Could you check a few things on this model? Use its own coordinates, in mm. A direction names the side the tool comes from. Coordinates: 2 decimals unless noted, no trailing zeros. Write each loop counter-clockwise with the first axis right and the second up, starting at its lowest first coordinate (ties: lowest second). Pieces come first, ordered by that corner, then holes. Notation, with made-up numbers: (-9.75, -6) - (44.25, -6) arc R28 ccw to (44.25, 12) - close; hole circle Ø2 at (2, 24.5). An arc over 180 degrees is marked (long way). Write item = value, one per line. Start each with the question number.
```python
from build123d import *

# Parameters (mm, degrees)
SKETCH1_W           = 57.5
SKETCH1_H           = 78
BOSS_EXTRUDE1_DEPTH = 30
SKETCH2_W           = 48.5
SKETCH2_H           = 26
CUT_EXTRUDE1_DEPTH  = 76
SKETCH3_R           = 2
SKETCH3_R_2         = 1
CUT_EXTRUDE2_DEPTH  = 60.424849114


with BuildPart() as part:
    # Sketch1 → Boss-Extrude1 (new body)
    with BuildSketch(Plane(origin=(0, 0, 0), x_dir=(1, 0, 0), z_dir=(0, 1, 0))):
        with Locations((-4.848039216, 1.230392157)):
            Rectangle(SKETCH1_W, SKETCH1_H)
    extrude(amount=BOSS_EXTRUDE1_DEPTH)

    # Sketch2 → Cut-Extrude1 (cut)
    with BuildSketch(Plane.XY.offset(37.769607843)):
        with Locations((-4.848039216, 15)):
            Rectangle(SKETCH2_W, SKETCH2_H)
    extrude(amount=-CUT_EXTRUDE1_DEPTH, mode=Mode.SUBTRACT)

    # Sketch3 → Cut-Extrude2 (cut, through all)
    with BuildSketch(Plane(origin=(0, 2, 0), x_dir=(1, 0, 0), z_dir=(0, 1, 0))):
        with Locations(Location((15.401960784, -33.769607843, 0), (0, 0, 270))):
            Circle(SKETCH3_R)
        with Locations(Location((-25.098039216, 34.230392157, 0), (0, 0, 270))):
            Circle(SKETCH3_R_2)
        with Locations(Location((-25.098039216, -33.769607843, 0), (0, 0, 270))):
            Circle(SKETCH3_R)
    extrude(amount=-CUT_EXTRUDE2_DEPTH, mode=Mode.SUBTRACT)


solid = part.part
```
1) Thinking about a two-plate mould opening in Y: for faces 1 (the flat face through (23.902, 15, -1)), 2 (the flat face through (-5, 15, -38.23)), 3 (the flat face through (-5, 30, -2)), 4 (the flat face through (-5, 28, 0)), which applies, +Y half, -Y half, draft (parallel to the pull), parting line (faces both ways), or undercut?
2) Suppose I cut it at A-A on z = -12.5. Please give me the cut outline in (x, y).
3) Which directions (+Z, -Z, +X, -X, +Y, -Y) give clear straight access to the entire face, cutting with the end or side of a thin tool? Please do faces 5 (the flat face through (-5, 0, -2)), 6 (the flat face through (-29.098, 15, 0)), 7 (the cylindrical face through (-26, 1, -33.8)).
4) If I drill on probe 1 along Y at (x, z) = (-5, 29); probe 2 along X at (y, z) = (23, 8); probe 3 along Z at (x, y) = (18, 16.75), over which ranges is the centre line in solid material (lowest first)? Write a range as [from, to].
5) Suppose I cut it at C-C on x = -7. Please give me the cut outline in (y, z), plus the area to 3 significant figures.
6) Suppose I cut it at B-B on y = 11. Please give me the cut outline in (x, z).
7) For P1, Ø13, axis at x = -17, y = 10, coming from the +Z side, with a flat end and sliding along its axis, tell me the tip position at first contact or that it passes through.
Reply:
q1.face_1 = draft
q1.face_2 = undercut
q1.face_3 = +Y half
q1.face_4 = undercut
q2.outline = (-33.6, 0) - (23.9, 0) - (23.9, 30) - (-33.6, 30) - close; hole (-29.1, 2) - (19.4, 2) - (19.4, 28) - (-29.1, 28) - close
q3.face_5 = +Z, -Z, +X, -X, -Y
q3.face_6 = +Z
q3.face_7 = -Y
q4.probe_1 = [0, 2], [28, 30]
q4.probe_2 = [-33.6, -29.1], [19.4, 23.9]
q4.probe_3 = [-40.23, -38.23]
q5.outline = (0, -40.23) - (30, -40.23) - (30, 37.77) - (28, 37.77) - (28, -38.23) - (2, -38.23) - (2, 37.77) - (0, 37.77) - close
q5.area = 364 mm^2
q6.outline = (-33.6, -40.23) - (23.9, -40.23) - (23.9, 37.77) - (19.4, 37.77) - (19.4, -38.23) - (-29.1, -38.23) - (-29.1, 37.77) - (-33.6, 37.77) - close
q7.P1 = -38.23
